from build123d import *

# Parameters (mm, degrees)
CROQUIS1_W              = 4.5
CROQUIS1_H              = 2.5
SALIENTE_EXTRUIR1_DEPTH = 3
REDONDEO1_R             = 1
CROQUIS2_R              = 1.5
SALIENTE_EXTRUIR2_DEPTH = 3


with BuildPart() as part:
    # Croquis1 → Saliente-Extruir1 (new body)
    with BuildSketch(Plane(origin=(0, 0, 0), x_dir=(1, 0, 0), z_dir=(0, 1, 0))):
        Polygon((4.5, 0), (-4.5, 0), (-4.5, 7), (-2, 7), (-2, 22), (2, 22), (2, 7), (4.5, 7), align=None)
        with Locations((0, 3.75)):
            Rectangle(CROQUIS1_W, CROQUIS1_H, mode=Mode.SUBTRACT)
    extrude(amount=SALIENTE_EXTRUIR1_DEPTH)

    # Redondeo1
    redondeo1_edges = [part.edges().sort_by_distance(p)[0] for p in [
        (-4.5, 1.5, -7),
        (4.5, 1.5, -7),
        (4.5, 1.5, 0),
        (-4.5, 1.5, 0),
    ]]
    fillet(redondeo1_edges, radius=REDONDEO1_R)

    # Croquis2 → Saliente-Extruir2 (add)
    with BuildSketch(Plane(origin=(0, 0, -22), x_dir=(-1, 0, 0), z_dir=(0, 0, -1))):
        with Locations(Location((0, 1.5, 0), (0, 0, 270))):
            Circle(CROQUIS2_R)
    extrude(amount=SALIENTE_EXTRUIR2_DEPTH)


solid = part.part
Input: part model. Units: mm. Frame: model coordinates. A direction names the side the tool comes from. Coordinates: 2 decimals unless noted, no trailing zeros. Order: outer loops, then holes, each group sorted by start corner. A loop starts at its lowest first (then second) coordinate and runs counter-clockwise, first axis right, second up. Notation, with made-up numbers: M 61.5,31.5 L 94.5,31.5 A21 cw 94.5,57.5 Z; hole C 18,29.25 d3. An arc over 180 degrees is marked long. Write item = value, one per line. Start each with the question number.
(1) Section D-D on y = 0.35. Output: boundary loops of the cut face in (x, z), and give its area (3 significant figures).
(2) Pull-direction query (Z, two-part tool) for faces 1 (the cylindrical face through (4.199, 1.521, -0.285)), 2 (the flat face through (2.25, 1, -4)), 3 (the flat face through (2, 1, -15)), 4 (the flat face through (0, 1, -2.5)); classes: released by +Z, released by -Z, zero draft, split by the parting line, or undercut.
(3) First-contact query: P1, Ø0.8, axis at x = 3, y = 2, coming from the -Z side; P2, Ø1.5, axis at y = 1.5, z = -11, coming from the +X side; P3, Ø1.5, axis at y = 1.5, z = -13, coming from the -X side. Flat tips, straight axial feed; report the tip coordinate or a pass-through.
(4) Reachability of faces 5 (the flat face through (-2, 1, -14)), 6 (the flat face through (1.7, 1.5, -22)), 7 (the flat face through (-1.7, 1.5, -22)), 8 (the flat face through (3, 1, -7)), 9 (the flat face through (-2.25, 1, -4)) from +Z, -Z, +X, -X, +Y, -Y: full face, straight path, thin tool, end or side. Return the list, or none.
(5) Section C-C on z = -19.25. Output: boundary loops of the cut face in (x, y).
(6) Line query: line 1 along Z through (x, y) = (0, 1.4); line 2 along Z through (x, y) = (1.75, 0.65); line 3 along X through (y, z) = (1.05, -4). Output: solid intervals per line, ascending. Write a range as [from, to].
(7) Section B-B on x = -1. Output: boundary loops of the cut face in (y, z).
(8) Section A-A on y = 1.5. Output: boundary loops of the cut face in (x, z).
Result set:
q1.outline = M -4.5,-6 A1 ccw -3.5,-7 L -2,-7 L -2,-22 L -0.96,-22 L -0.96,-25 L 0.96,-25 L 0.96,-22 L 2,-22 L 2,-7 L 3.5,-7 A1 ccw 4.5,-6 L 4.5,-1 A1 ccw 3.5,0 L -3.5,0 A1 ccw -4.5,-1 Z; hole M -2.25,-5 L 2.25,-5 L 2.25,-2.5 L -2.25,-2.5 Z
q1.area = 117 mm²
q2.face_1 = released by +Z
q2.face_2 = undercut
q2.face_3 = zero draft
q2.face_4 = undercut
q3.P1 = -7
q3.P2 = 2
q3.P3 = -2
q4.face_5 = -Z, -X, +Y, -Y
q4.face_6 = -Z, +X
q4.face_7 = -Z, -X
q4.face_8 = -Z, +X, +Y, -Y
q4.face_9 = +Y, -Y
q5.outline = M -2,0 L 2,0 L 2,3 L -2,3 Z
q6.line_1 = [-25, -5], [-2.5, 0]
q6.line_2 = [-22, -5], [-2.5, 0]
q6.line_3 = [-4.5, -2.25], [2.25, 4.5]
q7.outline = M 0,-22 L 0.38,-22 L 0.38,-25 L 2.62,-25 L 2.62,-22 L 3,-22 L 3,-5 L 0,-5 Z; M 0,-2.5 L 3,-2.5 L 3,0 L 0,0 Z
q8.outline = M -4.5,-6 A1 ccw -3.5,-7 L -2,-7 L -2,-22 L -1.5,-22 L -1.5,-25 L 1.5,-25 L 1.5,-22 L 2,-22 L 2,-7 L 3.5,-7 A1 ccw 4.5,-6 L 4.5,-1 A1 ccw 3.5,0 L -3.5,0 A1 ccw -4.5,-1 Z; hole M -2.25,-5 L 2.25,-5 L 2.25,-2.5 L -2.25,-2.5 Z
